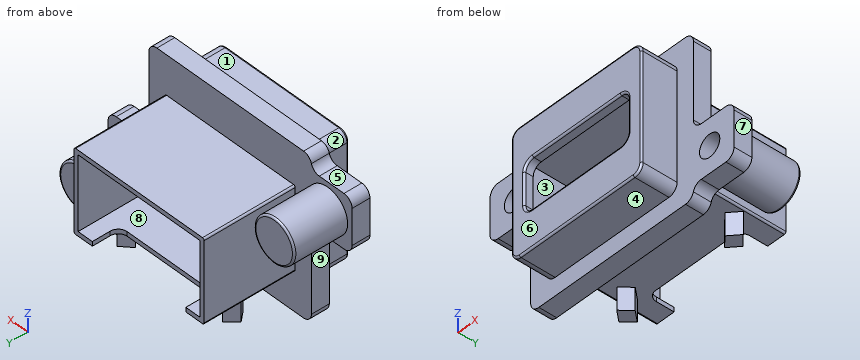
```python
from build123d import *

# Parameters (mm, degrees)
PAD_DEPTH       = 2
PAD001_DEPTH    = 4
PAD002_DEPTH    = 12.2
SKETCH003_W     = 15
SKETCH003_H     = 8.28
POCKET_DEPTH    = 15.2
SKETCH004_R     = 2.45
PAD003_DEPTH    = 8
SKETCH005_R     = 1.25
POCKET001_DEPTH = 5.5
POCKET002_DEPTH = 4.001
PAD004_DEPTH    = 2.5
POCKET003_DEPTH = 1
FILLET_R        = 0.2


with BuildPart() as part:
    # Sketch → Pad (new body)
    with BuildSketch(Plane.XZ):
        with BuildLine():
            Line((9, 13.64), (-9.031757, 13.64))
            ThreePointArc((-9.031757, 13.64), (-9.644125, 13.430572), (-10, 12.890009))
            ThreePointArc((-10.968248, 12.14), (-10.355872, 12.349434), (-10, 12.890009))
            Line((-10.968248, 12.14), (-14, 12.14))
            ThreePointArc((-14, 12.14), (-14.707107, 11.847107), (-15, 11.14))
            Line((-15, 11.14), (-15, 7.14))
            ThreePointArc((-15, 7.14), (-14.707107, 6.432893), (-14, 6.14))
            Line((-14, 6.14), (-11, 6.14))
            ThreePointArc((-10, 5.14), (-10.292893, 5.847107), (-11, 6.14))
            Line((-10, 5.14), (-10, -3.36))
            ThreePointArc((-10, -3.36), (-9.707107, -4.067107), (-9, -4.36))
            Line((-9, -4.36), (9.031755, -4.36))
            ThreePointArc((9.031755, -4.36), (9.644126, -4.150571), (10, -3.610004))
            ThreePointArc((10.968247, -2.86), (10.355873, -3.069432), (10, -3.610004))
            Line((10.968247, -2.86), (14, -2.86))
            ThreePointArc((14, -2.86), (14.707107, -2.567107), (15, -1.86))
            Line((15, -1.86), (15, 2.14))
            ThreePointArc((15, 2.14), (14.707107, 2.847107), (14, 3.14))
            Line((14, 3.14), (11, 3.14))
            ThreePointArc((10, 4.14), (10.292893, 3.432893), (11, 3.14))
            Line((10, 4.14), (10, 12.64))
            ThreePointArc((10, 12.64), (9.707107, 13.347107), (9, 13.64))
        make_face()
    extrude(amount=-PAD_DEPTH)

    # Sketch001 → Pad001 (join)
    with BuildSketch(Plane.XZ):
        with BuildLine():
            Line((-7, 11.64), (7, 11.64))
            ThreePointArc((8, 10.64), (7.707107, 11.347107), (7, 11.64))
            Line((8, 10.64), (8, -1.36))
            ThreePointArc((7, -2.36), (7.707107, -2.067107), (8, -1.36))
            Line((7, -2.36), (-7, -2.36))
            ThreePointArc((-8, -1.36), (-7.707107, -2.067107), (-7, -2.36))
            Line((-8, -1.36), (-8, 10.64))
            ThreePointArc((-7, 11.64), (-7.707107, 11.347107), (-8, 10.64))
        make_face()
    extrude(amount=PAD001_DEPTH)

    # Sketch002 → Pad002 (join)
    with BuildSketch(Plane.XZ):
        with BuildLine():
            Line((-7.8, 0), (7.8, 0))
            ThreePointArc((7.8, 0), (7.941421, 0.058579), (8, 0.2))
            Line((8, 0.2), (8, 9.08))
            ThreePointArc((8, 9.08), (7.941421, 9.221421), (7.8, 9.28))
            Line((7.8, 9.28), (-7.8, 9.28))
            ThreePointArc((-7.8, 9.28), (-7.941421, 9.221421), (-8, 9.08))
            Line((-8, 9.08), (-8, 0.2))
            ThreePointArc((-8, 0.2), (-7.941421, 0.058579), (-7.8, 0))
        make_face()
    extrude(amount=-PAD002_DEPTH)

    # Sketch003 → Pocket (cut)
    with BuildSketch(Plane.XZ.offset(-12.2)):
        with Locations((0, 4.64)):
            Rectangle(SKETCH003_W, SKETCH003_H)
    extrude(amount=POCKET_DEPTH, mode=Mode.SUBTRACT)

    # Sketch004 → Pad003 (join)
    with BuildSketch(Plane.XZ):
        with Locations((-12, 9.14)):
            Circle(SKETCH004_R)
        with Locations((12, 0.14)):
            Circle(SKETCH004_R)
    extrude(amount=-PAD003_DEPTH)

    # Sketch005 → Pocket001 (cut)
    with BuildSketch(Plane.XZ):
        with Locations((-12, 9.14)):
            Circle(SKETCH005_R)
        with Locations((12, 0.14)):
            Circle(SKETCH005_R)
    extrude(amount=-POCKET001_DEPTH, mode=Mode.SUBTRACT)

    # Sketch006 → Pocket002 (cut, through all)
    with BuildSketch(Plane.XZ):
        with BuildLine():
            Line((-5.4, 7.44), (5.4, 7.44))
            ThreePointArc((6.4, 6.44), (6.107107, 7.147107), (5.4, 7.44))
            Line((6.4, 6.44), (6.4, 2.84))
            ThreePointArc((5.4, 1.84), (6.107107, 2.132893), (6.4, 2.84))
            Line((5.4, 1.84), (-5.4, 1.84))
            ThreePointArc((-6.4, 2.84), (-6.107107, 2.132893), (-5.4, 1.84))
            Line((-6.4, 2.84), (-6.4, 6.44))
            ThreePointArc((-5.4, 7.44), (-6.107107, 7.147107), (-6.4, 6.44))
        make_face()
    extrude(amount=POCKET002_DEPTH, mode=Mode.SUBTRACT)

    # Sketch007 → Pad004 (join)
    with BuildSketch(Plane.XY):
        Polygon((-6.57, 8.82), (-7.57, 7.67), (-6.57, 6.52), (-5.57, 7.67), align=None)
        Polygon((6.57, 8.67), (5.42, 7.67), (6.57, 6.67), (7.72, 7.67), align=None)
    extrude(amount=-PAD004_DEPTH)

    # Sketch008 → Pocket003 (cut)
    with BuildSketch(Plane.XY):
        with BuildLine():
            Line((-5.75, 12.2), (5.75, 12.2))
            Line((5.75, 12.2), (5.75, 10.2))
            ThreePointArc((4.75, 9.2), (5.457107, 9.492893), (5.75, 10.2))
            Line((4.75, 9.2), (-4.75, 9.2))
            ThreePointArc((-5.75, 10.2), (-5.457107, 9.492893), (-4.75, 9.2))
            Line((-5.75, 10.2), (-5.75, 12.2))
        make_face()
    extrude(amount=POCKET003_DEPTH, mode=Mode.SUBTRACT)

    # Fillet
    fillet_edges = [part.edges().sort_by_distance(p)[0] for p in [
        (0, -4, 11.64),
        (0, -4, 7.44),
        (-14.45, 8, 9.14),
        (9.55, 8, 0.14),
    ]]
    fillet(fillet_edges, radius=FILLET_R)


solid = part.part
```
Source: CAD feature listing. Evaluate the final solid. Frame: model axes, mm. Face numbers are marked on the shaded views. A direction names the side the tool comes from. Coordinates: 2 decimals unless noted, no trailing zeros. Write each loop counter-clockwise with the first axis right and the second up, starting at its lowest first coordinate (ties: lowest second). Pieces come first, ordered by that corner, then holes. Notation, with made-up numbers: (65.5, 23.25) - (112.5, 23.25) arc R30 cw to (112.5, 53.25) - close; hole circle Ø6 at (-2, -33.5). An arc over 180 degrees is marked (long way). Answer as a JSON object with one key per item and string values.
Q1. First-contact query: pin 1 Ø6 at (y, z) = (4.5, 11) entering from -X; pin 2 Ø2 at (x, y) = (2.5, 9.5) entering from +Z; pin 3 Ø2 at (x, y) = (12, 0.5) entering from -Z; pin 4 Ø7.5 at (x, y) = (2.5, 6) entering from -Z. Flat tips, straight axial feed; report the tip coordinate or a pass-through.
Ans:
{"pin 1": "stops at x = -15", "pin 2": "stops at z = 9.28", "pin 3": "stops at z = -2.86", "pin 4": "stops at z = -2.5"}
Q2. Section query C-C, the plane y = 11. Output: boundary loops of the cut face in (x, z), plus the area to 3 significant figures.
Ans:
{"outline": "(-8, 0.2) arc R0.2 ccw to (-7.8, 0) - (-5.75, 0) - (-5.75, 0.5) - (-7.5, 0.5) - (-7.5, 8.78) - (7.5, 8.78) - (7.5, 0.5) - (5.75, 0.5) - (5.75, 0) - (7.8, 0) arc R0.2 ccw to (8, 0.2) - (8, 9.08) arc R0.2 ccw to (7.8, 9.28) - (-7.8, 9.28) arc R0.2 ccw to (-8, 9.08) - close", "area": "18.5 mm2"}
Q3. Section query B-B, the plane x = -12. Output: boundary loops of the cut face in (y, z).
Ans:
{"outline": "(0, 6.14) - (2, 6.14) - (2, 6.69) - (7.8, 6.69) arc R0.2 ccw to (8, 6.89) - (8, 11.39) arc R0.2 ccw to (7.8, 11.59) - (2, 11.59) - (2, 12.14) - (0, 12.14) - (0, 10.39) - (5.5, 10.39) - (5.5, 7.89) - (0, 7.89) - close"}
Q4. Material intervals for line 1 (X direction, y = 5.75, z = 9); line 2 (Z direction, x = 5.5, y = 6.75); line 3 (X direction, y = 1, z = 4.25), sorted ascending. Write a range as [from, to].
Ans:
{"line 1": "x = [-14.45, -9.55], [-8, 8]", "line 2": "z = [0, 0.5], [8.78, 9.28]", "line 3": "x = [-10, -7.5], [7.5, 10]"}
Q5. Draft query along X for the marked faces 6, 7, 8 and 9. Return one class per face: released by +X, released by -X, zero draft, split by the parting line, or undercut.
Ans:
{"face 6": "zero draft", "face 7": "released by +X", "face 8": "undercut", "face 9": "released by -X"}
Q6. Set-up query: the marked faces 1, 2, 3, 4 and 5. Return all of +Z, -Z, +X, -X, +Y, -Y with unobstructed straight access to the full face (end or side cutting, diameter ignored); none if empty.
Ans:
{"face 1": "+Z, +X, -X, -Y", "face 2": "+Z, -X, -Y", "face 3": "+Y", "face 4": "-Z, +X, -X, -Y", "face 5": "+Z, -X, +Y, -Y"}
Q7. Section query A-A, the plane y = 0.5. Output: boundary loops of the cut face in (x, z), plus the area to 3 significant figures.
Ans:
{"outline": "(-15, 7.14) arc R1 ccw to (-14, 6.14) - (-11, 6.14) arc R1 cw to (-10, 5.14) - (-10, -3.36) arc R1 ccw to (-9, -4.36) - (9.03, -4.36) arc R1 ccw to (10, -3.61) arc R1 cw to (10.97, -2.86) - (14, -2.86) arc R1 ccw to (15, -1.86) - (15, 2.14) arc R1 ccw to (14, 3.14) - (11, 3.14) arc R1 cw to (10, 4.14) - (10, 12.64) arc R1 ccw to (9, 13.64) - (-9.03, 13.64) arc R1 ccw to (-10, 12.89) arc R1 cw to (-10.97, 12.14) - (-14, 12.14) arc R1 ccw to (-15, 11.14) - close; hole circle Ø2.5 at (-12, 9.14); hole (-7.5, 0.5) - (7.5, 0.5) - (7.5, 8.78) - (-7.5, 8.78) - close; hole circle Ø2.5 at (12, 0.14)", "area": "285 mm2"}
